from build123d import *


with BuildPart() as part:
    # Sketch → Revolution (revolve)
    with BuildSketch(Plane.XZ):
        with BuildLine():
            Line((8.5, 94), (9.5, 94))
            Line((9.5, 94), (9.5, 95))
            Line((9.5, 95), (8.5, 95))
            Line((8.5, 95), (8.5, 100))
            Line((8.5, 100), (7.5, 100))
            Line((7.5, 100), (7.5, 13.555724))
            Line((7.5, 13.555724), (0, 4.617572))
            Line((0, 4.173296), (0, 4.617572))
            ThreePointArc((0, 4.173296), (0.845237, 4.36068), (1.532089, 4.88772))
            Line((1.532089, 4.88772), (7.5, 12))
            Line((7.5, 12), (7.5, 0))
            Line((7.5, 0), (8.5, 0))
            Line((8.5, 0), (8.5, 94))
        make_face()
    revolve(axis=Axis((0, 0, 0), (0, 0, 1)))


solid = part.part
Can you work these out from the model? Positions are in its coordinate system, mm. A direction names the side the tool comes from. Coordinates: 2 decimals unless noted, no trailing zeros. Loops run counter-clockwise (first coordinate to the right, second up) from the corner with the lowest first, then second, coordinate; pieces in that order, holes last. Notation, with made-up numbers: (27.25, 85.25) - (67.25, 85.25) arc R6 cw to (67.25, 91.25) - close; hole circle Ø11 at (28, 8.25). An arc over 180 degrees is marked (long way). Put each result on its own line as item: value. Start each with the question number.
Item 1: If I drill on line 1 along Y through (x, z) = (0, 58); line 2 along Y through (x, z) = (6.5, 6.5); line 3 along X through (y, z) = (1, 7.5), over which ranges is the centre line in solid material (lowest first)?
Item 2: If we mould it in two halves opening along Y, with no side actions, what happens to faces 4 (the face through (0, -8, 0)), 5 (the face through (4.57, 7.167, 47.658)), 6 (the face through (1.94, 0.61, 7.04))? For each: +Y half, -Y half, draft (parallel to the pull), parting line (faces both ways), or undercut.
Item 3: For pin 1 (1 mm diameter, centred on x = -4, y = -5, fed in from +Z); pin 2 (9 mm diameter, centred on x = 0, y = 0, fed in from -Z); pin 3 (1.5 mm diameter, centred on y = -3.5, z = 29, fed in from -X), each with a flat end and sliding along its axis, tell me the tip position at first contact or that it passes through.
Item 4: Suppose I cut it at A-A (z = 56). Please give me the cut outline in (x, y).
Item 5: Which directions (+Z, -Z, +X, -X, +Y, -Y) give clear straight access to the entire face, cutting with the end or side of a thin tool? Please do faces 1 (the face through (-7.493, 0.33, 56.173)), 2 (the face through (2.2, -8.4, 94)), 3 (the face through (4.38, -8.43, 94.51)).
Here are the results:
1. line 1: -8.5 to -7.5, 7.5 to 8.5
1. line 2: -5.48 to -3.74, 3.74 to 5.48
1. line 3: -8.44 to -7.43, -3.59 to -2.2, 2.2 to 3.59, 7.43 to 8.44
2. face 4: draft
2. face 5: parting line
2. face 6: undercut
3. pin 1: z = 12.84
3. pin 2: z = 4.17
3. pin 3: x = -8.04
4. outline: circle Ø17 at (0, 0); hole circle Ø15 at (0, 0)
5. face 1: +Z
5. face 2: -Z
5. face 3: +Z, -Z
